Geometry: final body of the model. Coordinates: model frame, mm. A direction names the side the tool comes from. Give positions to 0.01 mm unless a question says otherwise; leave off trailing zeros. Write each loop counter-clockwise with the first axis right and the second up, starting at its lowest first coordinate (ties: lowest second). Pieces come first, ordered by that corner, then holes.
Q1. Line query: line 1 (X direction, y = 1.25, z = -6); line 2 (Z direction, x = -5, y = 1); line 3 (Z direction, x = 6.5, y = 0.7). Output: solid intervals per line, ascending.
Q2. Mould query, pull axis Z, two halves, no side actions, for faces 3 (the cylindrical face through (6.93, 1.48, 9.4)), 4 (the flat face through (5.5, 1, -6)), 5 (the cylindrical face through (6.9, 1.48, -9.43)), 6 (the flat face through (0, 0, 0)). Classes: +Z half, -Z half, draft (parallel to the pull), parting line (faces both ways), or undercut.
Q3. Section A-A (x = 2). Return the cut outline in (y, z).
Q4. Section B-B (z = 4.75). Return the cut outline in (x, y), plus the area to 3 significant figures.
Q5. Section C-C (y = 2.1). Return the cut outline in (x, z), plus the area to 3 significant figures.
Q6. Reachability of faces 1 (the cylindrical face through (-6.9, 1.48, 9.43)), 2 (the flat face through (3, 1, -7.5)) from +Z, -Z, +X, -X, +Y, -Y: full face, straight path, thin tool, end or side. Return the list, or none.
Autodesk Inventor part; units mm, degrees
ref_plane "YZ Plane" through (0, 0, 0) normal (1, 0, 0) x (0, 1, 0)
ref_plane "XZ Plane" through (0, 0, 0) normal (0, 1, 0) x (-1, 0, 0)
ref_plane "XY Plane" through (0, 0, 0) normal (0, 0, 1) x (1, 0, 0)
sketch "Sketch1" plane through (0, 0, 0) normal (0, 1, 0) x (-1, 0, 0)
  line L0 (5.5, 10) -> (-5.5, 10)
  line L1 (-7.5, 8) -> (-7.5, -8)
  line L2 (-5.5, -10) -> (5.5, -10)
  line L3 (7.5, -8) -> (7.5, 8)
  line L4 (7.5, 10) -> (-7.5, -10) construction
  line L5 (-7.5, 10) -> (7.5, -10) construction
  arc A0 (7.5, 8) -> (5.5, 10) centre (5.5, 8) ccw
  arc A1 (-5.5, 10) -> (-7.5, 8) centre (-5.5, 8) ccw
  arc A2 (-7.5, -8) -> (-5.5, -10) centre (-5.5, -8) ccw
  arc A3 (5.5, -10) -> (7.5, -8) centre (5.5, -8) ccw
  line L6 (5.5, 7.5) -> (1, 7.5)
  line L7 (1, 7.5) -> (1, 4.5)
  line L8 (1, 4.5) -> (5.5, 4.5)
  line L9 (5.5, 4.5) -> (5.5, 7.5)
  line L10 (0, 0) -> (2.8076, 0) construction
  line L11 (0, 0) -> (0, 2.1917) construction
  line L12 (5.5, -7.5) -> (1, -7.5)
  line L13 (1, -7.5) -> (1, -4.5)
  line L14 (1, -4.5) -> (5.5, -4.5)
  line L15 (5.5, -4.5) -> (5.5, -7.5)
  line L16 (-7.5, 10) -> (7.5, -10) construction
  line L17 (-5.5, 7.5) -> (-1, 7.5)
  line L18 (-1, 7.5) -> (-1, 4.5)
  line L19 (-1, 4.5) -> (-5.5, 4.5)
  line L20 (-5.5, 4.5) -> (-5.5, 7.5)
  line L21 (-5.5, -4.5) -> (-5.5, -7.5)
  line L22 (-5.5, -7.5) -> (-1, -7.5)
  line L23 (-1, -7.5) -> (-1, -4.5)
  line L24 (-1, -4.5) -> (-5.5, -4.5)
  point P0 (-5.5, 8)
  point P1 (-5.5, -8)
  dimension "d2" = 2
  dimension "d3" = 2
  dimension "d4" = 16
  dimension "d5" = 11
  dimension "d9" = 4.5
  dimension "d10" = 3
  dimension "d11" = 2.5
  dimension "d12" = 2
extrude "Extrusion1" add sketch "Sketch1" along normal blind 3
properties part number "Hinge_Base"
Computed:
1. line 1: x = -7.5 to -5.5, -1 to 1, 5.5 to 7.5
1. line 2: z = -10 to -7.5, -4.5 to 4.5, 7.5 to 10
1. line 3: z = -9.73 to 9.73
2. face 3: +Z half
2. face 4: undercut
2. face 5: -Z half
2. face 6: draft
3. outline: (0, -10) - (3, -10) - (3, -7.5) - (0, -7.5) - close; (0, -4.5) - (3, -4.5) - (3, 4.5) - (0, 4.5) - close; (0, 7.5) - (3, 7.5) - (3, 10) - (0, 10) - close
4. outline: (-7.5, 0) - (-5.5, 0) - (-5.5, 3) - (-7.5, 3) - close; (-1, 0) - (1, 0) - (1, 3) - (-1, 3) - close; (5.5, 0) - (7.5, 0) - (7.5, 3) - (5.5, 3) - close
4. area: 18.0 mm2
5. outline: (-7.5, -8) arc R2 ccw to (-5.5, -10) - (5.5, -10) arc R2 ccw to (7.5, -8) - (7.5, 8) arc R2 ccw to (5.5, 10) - (-5.5, 10) arc R2 ccw to (-7.5, 8) - close; hole (-5.5, -7.5) - (-1, -7.5) - (-1, -4.5) - (-5.5, -4.5) - close; hole (-5.5, 4.5) - (-1, 4.5) - (-1, 7.5) - (-5.5, 7.5) - close; hole (1, -7.5) - (5.5, -7.5) - (5.5, -4.5) - (1, -4.5) - close; hole (1, 4.5) - (5.5, 4.5) - (5.5, 7.5) - (1, 7.5) - close
5. area: 243 mm2
6. face 1: +Z, -X, +Y, -Y
6. face 2: +Y, -Y
